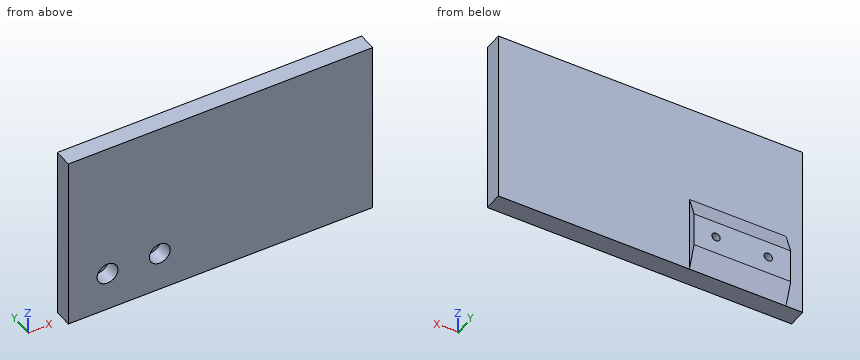
from build123d import *

# Parameters (mm, degrees)
F0_W     = 116.5554597974
F0_H     = 67.673869431
F1_DEPTH = 7
F4_START = -6.4
F4_DEPTH = 37
F2_R     = 1.6
F5_DEPTH = 10.001
F2_R_2   = 4
F6_DEPTH = 6


with BuildPart() as f1:
    # F0 (on Front) → F1 (new body)
    with BuildSketch(Plane.XZ):
        with Locations((58.2777298987, 33.8369347155)):
            Rectangle(F0_W, F0_H)
    extrude(amount=F1_DEPTH)

    # F3 (on face) → F4 (join)
    with BuildSketch(Plane(origin=(0, 0, 0), x_dir=(0, -1, 0), z_dir=(-1, 0, 0)).offset(F4_START)):
        Polygon((-3, 8.2424322584), (0, 0), (0, 29.4848645167), (-3, 21.2424322584), align=None)
    extrude(amount=-F4_DEPTH)

    # F2 (on face) → F5 (cut, through all)
    with BuildSketch(Plane.XZ.offset(7)):
        with Locations((15, 15)):
            Circle(F2_R)
        with Locations((35, 15)):
            Circle(F2_R)
    extrude(amount=-F5_DEPTH, mode=Mode.SUBTRACT)

    # F2 (on face) → F6 (cut)
    with BuildSketch(Plane.XZ.offset(7)):
        with Locations((15, 15)):
            Circle(F2_R_2)
        with Locations((15, 15)):
            Circle(F2_R, mode=Mode.SUBTRACT)
        with Locations((35, 15)):
            Circle(F2_R_2)
        with Locations((35, 15)):
            Circle(F2_R, mode=Mode.SUBTRACT)
    extrude(amount=-F6_DEPTH, mode=Mode.SUBTRACT)


solid = f1.part
Model file for the job. Use its own axes, mm. Round coordinates to 2 decimals unless told otherwise and drop trailing zeros. Order: outer loops, then holes, each group sorted by start corner. A loop starts at its lowest first (then second) coordinate and runs counter-clockwise, first axis right, second up.
(1) Band-saw the part on D-D (z = 63). List the corners of the cut face in (x, y), then the cut area to 3 significant figures.
(2) Band-saw the part on C-C (y = 1.5). List the corners of the cut face in (x, z).
(3) Band-saw the part on A-A (x = 35). List the corners of the cut face in (y, z).
(4) Pin check, flat tips, straight feed: pin 1 (3 mm diameter, centred on x = 35, z = 15, fed in from -Y); pin 2 (6.5 mm diameter, centred on x = 15, z = 15, fed in from +Y); pin 3 (1.5 mm diameter, centred on y = 1, z = 13.5, fed in from +X); pin 4 (5 mm diameter, centred on x = 29.5, z = 48, fed in from +Y). Stop position of each tip, or through.
(5) Drill centre lines: line 1 (Z direction, x = 35, y = -2.6); line 2 (X direction, y = -4.5, z = 17); line 3 (Y direction, x = 86.5, z = 20.5). Where is each one in solid material? Low to high.
(6) Band-saw the part on B-B (z = 15). List the corners of the cut face in (x, y).
Verdict:
1. outline: (0, -7) - (116.56, -7) - (116.56, 0) - (0, 0) - close
1. area: 816 mm2
2. outline: (6.4, 4.12) - (43.4, 4.12) - (43.4, 25.36) - (6.4, 25.36) - close; hole circle Ø3.2 at (15, 15); hole circle Ø3.2 at (35, 15)
3. outline: (-7, 0) - (0, 0) - (3, 8.24) - (3, 13.4) - (-1, 13.4) - (-1, 11) - (-7, 11) - close; (-7, 19) - (-1, 19) - (-1, 16.6) - (3, 16.6) - (3, 21.24) - (0, 29.48) - (0, 67.67) - (-7, 67.67) - close
4. pin 1: passes through
4. pin 2: stops at y = 3
4. pin 3: stops at x = 43.4
4. pin 4: stops at y = 0
5. line 1: z = 0 to 11, 19 to 67.67
5. line 2: x = 0 to 11.54, 18.46 to 31.54, 38.46 to 116.56
5. line 3: y = -7 to 0
6. outline: (0, -7) - (11, -7) - (11, -1) - (13.4, -1) - (13.4, 3) - (6.4, 3) - (6.4, 0) - (0, 0) - close; (16.6, -1) - (19, -1) - (19, -7) - (31, -7) - (31, -1) - (33.4, -1) - (33.4, 3) - (16.6, 3) - close; (36.6, -1) - (39, -1) - (39, -7) - (116.56, -7) - (116.56, 0) - (43.4, 0) - (43.4, 3) - (36.6, 3) - close
